Check sheet for the modelled part. Datum: model origin and axes. Units: mm. Give positions to 0.01 mm unless a question says otherwise; leave off trailing zeros. Loops run counter-clockwise (first coordinate to the right, second up) from the corner with the lowest first, then second, coordinate; pieces in that order, holes last. Notation, with made-up numbers: (57.25, 38.5) - (74.25, 38.5) arc R28 cw to (74.25, 70.5) - close; hole circle Ø4 at (68, 3). An arc over 180 degrees is marked (long way). Answer in a Markdown table with one row per item. Add a question column.
(1) Sectioned sample at B-B on x = 21. Enter the section's corners in (y, z), then the cut area to 4 significant figures.
(2) Thickness scan on L1, parallel to X at y = 5, z = 0; L2, parallel to X at y = 8.3, z = -35; L3, parallel to X at y = 3.5, z = -35. Record the ranges inside material, lowest first.
(3) Go/stop test with flat-tipped pins: P1, Ø11.5, axis at x = 36, z = -35, coming from the -Y side; P2, Ø1, axis at x = -56.5, y = 5.5, coming from the +Z side; P3, Ø1, axis at y = 6.5, z = 29, coming from the -X side; P4, Ø2, axis at y = 2.5, z = -24.5, coming from the -X side. Record where each tip stops, or that it passes through.
(4) Sectioned sample at A-A on z = 0. Enter the section's corners in (x, y).
(5) Sectioned sample at D-D on y = 7. State how many separate pieces and enclosed holes the cut face has, then the cut area to 3 significant figures.
(6) Sectioned sample at C-C on z = -35. Enter the section's corners in (x, y), then the cut area to 3 significant figures.
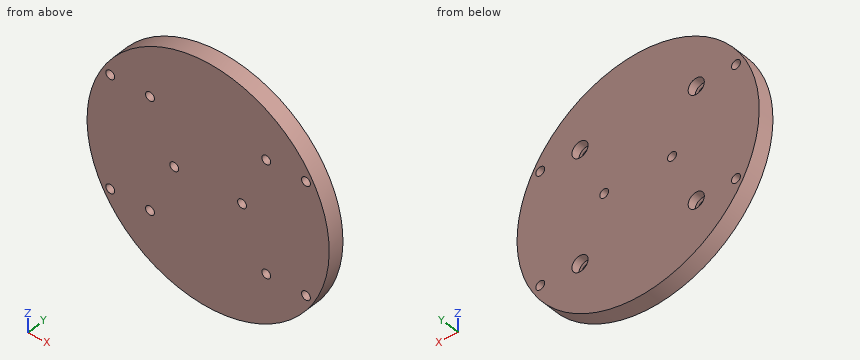
from build123d import *

# Parameters (mm, degrees)
SKETCH_1_R          = 75
EXTRUDE_1_DEPTH     = 10
SKETCH_2_R          = 2.75
CUT_EXTRUDE_1_DEPTH = 27
SKETCH_3_R          = 5
CUT_EXTRUDE_2_DEPTH = 5


with BuildPart() as part:
    # 草图1 → 凸台-拉伸1 (new body)
    with BuildSketch(Plane(origin=(0, 0, 0), x_dir=(1, 0, 0), z_dir=(0, 1, 0))):
        with Locations(Location((0, 0, 0), (0, 0, 270))):
            Circle(SKETCH_1_R)
    extrude(amount=EXTRUDE_1_DEPTH)

    # 草图2 → 切除-拉伸1 (cut)
    with BuildSketch(Plane(origin=(0, 10, 0), x_dir=(1, 0, 0), z_dir=(0, 1, 0))):
        with Locations(Location((21, 0, 0), (0, 0, 270))):
            Circle(SKETCH_2_R)
        with Locations(Location((-21, 0, 0), (0, 0, 270))):
            Circle(SKETCH_2_R)
        with Locations(Location((36, 35, 0), (0, 0, 270))):
            Circle(SKETCH_2_R)
        with Locations(Location((36, -35, 0), (0, 0, 270))):
            Circle(SKETCH_2_R)
        with Locations(Location((-36, -35, 0), (0, 0, 270))):
            Circle(SKETCH_2_R)
        with Locations(Location((-36, 35, 0), (0, 0, 270))):
            Circle(SKETCH_2_R)
        with Locations(Location((60.621778265, 35, 0), (0, 0, 270))):
            Circle(SKETCH_2_R)
        with Locations(Location((60.621778265, -35, 0), (0, 0, 270))):
            Circle(SKETCH_2_R)
        with Locations(Location((-60.621778265, -35, 0), (0, 0, 270))):
            Circle(SKETCH_2_R)
        with Locations(Location((-60.621778265, 35, 0), (0, 0, 270))):
            Circle(SKETCH_2_R)
    extrude(amount=-CUT_EXTRUDE_1_DEPTH, mode=Mode.SUBTRACT)

    # 草图3 → 切除-拉伸2 (cut)
    with BuildSketch(Plane(origin=(0, 10, 0), x_dir=(1, 0, 0), z_dir=(0, 1, 0))):
        with Locations(Location((36, 35, 0), (0, 0, 270))):
            Circle(SKETCH_3_R)
        with Locations(Location((36, -35, 0), (0, 0, 270))):
            Circle(SKETCH_3_R)
        with Locations(Location((-36, -35, 0), (0, 0, 270))):
            Circle(SKETCH_3_R)
        with Locations(Location((-36, 35, 0), (0, 0, 270))):
            Circle(SKETCH_3_R)
    extrude(amount=-CUT_EXTRUDE_2_DEPTH, mode=Mode.SUBTRACT)


solid = part.part
Reply:
| question | item | result |
|---|---|---|
| 1 | outline | (0, -72) - (10, -72) - (10, -2.75) - (0, -2.75) - close; (0, 2.75) - (10, 2.75) - (10, 72) - (0, 72) - close |
| 1 | area | 1,385 mm^2 |
| 2 | L1 | -75 to -23.75, -18.25 to 18.25, 23.75 to 75 |
| 2 | L2 | -66.33 to -63.37, -57.87 to -41, -31 to 31, 41 to 57.87, 63.37 to 66.33 |
| 2 | L3 | -66.33 to -63.37, -57.87 to -38.75, -33.25 to 33.25, 38.75 to 57.87, 63.37 to 66.33 |
| 3 | P1 | y = 0 |
| 3 | P2 | z = 49.89 |
| 3 | P3 | x = -69.37 |
| 3 | P4 | x = -71.22 |
| 4 | outline | (-75, 0) - (-23.75, 0) - (-23.75, 10) - (-75, 10) - close; (-18.25, 0) - (18.25, 0) - (18.25, 10) - (-18.25, 10) - close; (23.75, 0) - (75, 0) - (75, 10) - (23.75, 10) - close |
| 5 | separate pieces | 1 |
| 5 | enclosed holes | 10 |
| 5 | area | 17,200 mm^2 |
| 6 | outline | (-66.33, 0) - (-63.37, 0) - (-63.37, 10) - (-66.33, 10) - close; (-57.87, 0) - (-38.75, 0) - (-38.75, 5) - (-41, 5) - (-41, 10) - (-57.87, 10) - close; (-33.25, 0) - (33.25, 0) - (33.25, 5) - (31, 5) - (31, 10) - (-31, 10) - (-31, 5) - (-33.25, 5) - close; (38.75, 0) - (57.87, 0) - (57.87, 10) - (41, 10) - (41, 5) - (38.75, 5) - close; (63.37, 0) - (66.33, 0) - (66.33, 10) - (63.37, 10) - close |
| 6 | area | 1,060 mm^2 |
